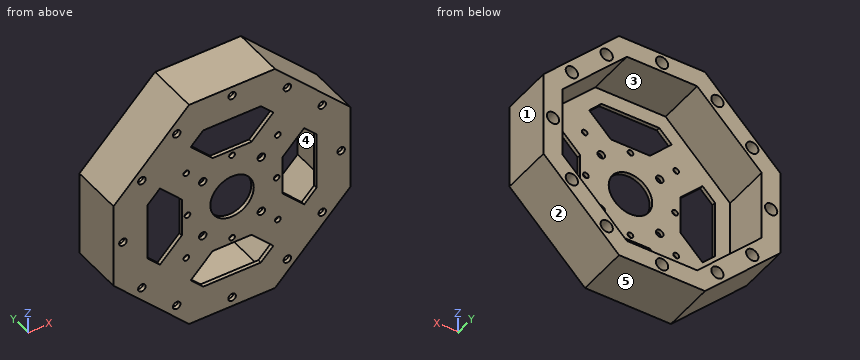
Autodesk Inventor part; units mm, degrees
ref_plane "YZ Plane" through (0, 0, 0) normal (1, 0, 0) x (0, 1, 0)
ref_plane "XZ Plane" through (0, 0, 0) normal (0, 1, 0) x (-1, 0, 0)
ref_plane "XY Plane" through (0, 0, 0) normal (0, 0, 1) x (1, 0, 0)
sketch "Sketch1" plane through (0, 0, 0) normal (0, 1, 0) x (-1, 0, 0)
  line L0 (0, 0) -> (0, 22.75)
  line L1 (40, 62.75) -> (0, 22.75)
  line L2 (40, 62.75) -> (85.5, 62.75)
  line L3 (85.5, 62.75) -> (125.5, 22.75)
  line L4 (125.5, 22.75) -> (125.5, 0)
  line L5 (0, 0) -> (0, -22.75)
  line L6 (40, -62.75) -> (0, -22.75)
  line L7 (40, -62.75) -> (85.5, -62.75)
  line L8 (85.5, -62.75) -> (125.5, -22.75)
  line L9 (125.5, -22.75) -> (125.5, 0)
  dimension "d0" = 22.75
  dimension "d3" = 45.5
  dimension "d4" = 135
extrude "Extrusion1" add sketch "Sketch1" along normal blind 2
sketch "Sketch2" plane through (0, 2, 0) normal (0, 1, 0) x (1, 0, 0)
  line L0 (-85.5, -62.75) -> (-40, -62.75)
  line L1 (-62.75, -62.75) -> (-62.75, 0)
  circle A0 centre (-62.75, 0) radius 11.5
  point P0 (0, 0)
  point P1 (-78.25, -15.5)
  point P2 (-47.25, -15.5)
  point P3 (-47.25, 15.5)
  point P4 (-78.25, 15.5)
  dimension "d7" = 23
extrude "Extrusion2" cut sketch "Sketch2" against normal blind 2
sketch "Sketch3" plane through (0, 2, 0) normal (0, 1, 0) x (1, 0, 0)
  circle A0 centre (-62.75, 0) radius 11.5
  point P0 (0, 0)
  point P1 (-78.25, -15.5)
  point P2 (-47.25, -15.5)
  point P3 (-47.25, 15.5)
  point P4 (-78.25, 15.5)
hole "Hole1" at (-78.25, 2, 15.5) at (-47.25, 2, 15.5) at (-47.25, 2, -15.5) at (-78.25, 2, -15.5) direction (0, -1, 0) diameter 4 depth 2 tip angle 118
sketch "Sketch4" plane through (0, 2, 0) normal (0, 1, 0) x (1, 0, 0)
  line L0 (-125.5, -22.75) -> (-85.5, -62.75)
  line L1 (-85.5, -62.75) -> (-125.5, -22.75)
  line L2 (-125.5, 22.75) -> (-125.5, -22.75)
  line L3 (-125.5, -22.75) -> (-125.5, 22.75)
  line L4 (-85.5, 62.75) -> (-125.5, 22.75)
  line L5 (-125.5, 22.75) -> (-85.5, 62.75)
  line L6 (-40, 62.75) -> (-85.5, 62.75)
  line L7 (-85.5, 62.75) -> (-40, 62.75)
  line L8 (0, -22.75) -> (0, 22.75)
  line L9 (-40, 62.75) -> (0, 22.75)
  line L10 (0, 22.75) -> (0, -22.75)
  line L11 (-40, -62.75) -> (0, -22.75)
  line L12 (0, -22.75) -> (-40, -62.75)
  line L13 (-85.5, -62.75) -> (-40, -62.75)
  line L14 (-40, -62.75) -> (-85.5, -62.75)
  circle A0 centre (-62.75, 0) radius 11.5
  point P0 (0, 0)
  point P1 (-62.75, -57.75)
  point P2 (-92.0542, -49.1247)
  point P3 (-110.5001, -30.6788)
  point P4 (-33.4458, -49.1247)
  point P5 (-14.9999, -30.6788)
  point P6 (-5, 0)
  point P7 (-120.5, 0)
  point P8 (-62.75, 57.75)
  point P9 (-92.0542, 49.1247)
  point P10 (-110.5001, 30.6788)
  point P11 (-33.4458, 49.1247)
  point P12 (-14.9999, 30.6788)
hole "Hole2" at (-62.75, 2, 57.75) at (-92.0542, 2, 49.1247) at (-110.5001, 2, 30.6788) at (-33.4458, 2, 49.1247) at (-14.9999, 2, 30.6788) at (-5, 2, 0) at (-120.5, 2, 0) at (-110.5001, 2, -30.6788) at (-92.0542, 2, -49.1247) at (-62.75, 2, -57.75) at (-33.4458, 2, -49.1247) at (-14.9999, 2, -30.6788) direction (0, -1, 0) diameter 4 depth 2 tip angle 118
sketch "Sketch5" plane through (0, 2, 0) normal (0, 1, 0) x (1, 0, 0)
  line L0 (-40, -62.75) -> (0, -22.75)
  line L1 (-85.5, -62.75) -> (-40, -62.75)
  line L2 (-40, -62.75) -> (-85.5, -62.75)
  line L3 (-125.5, 22.75) -> (-125.5, -22.75)
  line L4 (-85.5, -62.75) -> (-125.5, -22.75)
  line L5 (-125.5, -22.75) -> (-125.5, 22.75)
  line L6 (-85.5, 62.75) -> (-125.5, 22.75)
  line L7 (-125.5, 22.75) -> (-85.5, 62.75)
  line L8 (-40, 62.75) -> (-85.5, 62.75)
  line L9 (-85.5, 62.75) -> (-40, 62.75)
  line L10 (0, -22.75) -> (0, 22.75)
  line L11 (-40, 62.75) -> (0, 22.75)
  line L12 (0, 22.75) -> (0, -22.75)
  line L13 (0, -22.75) -> (-40, -62.75)
  line L14 (-81.3579, -52.75) -> (-44.1421, -52.75)
  line L15 (-10, -18.6079) -> (-10, 18.6079)
  line L16 (-44.1421, 52.75) -> (-81.3579, 52.75)
  line L17 (-115.5, 18.6079) -> (-115.5, -18.6079)
  line L18 (-49.1421, -18.6079) -> (-76.3579, -18.6079)
  line L19 (-81.3579, -13.6079) -> (-81.3579, 13.6079)
  line L20 (-76.3579, 18.6079) -> (-49.1421, 18.6079)
  line L21 (-44.1421, 13.6079) -> (-44.1421, -13.6079)
  line L22 (-44.1421, -13.6079) -> (-24.5711, -33.1789)
  line L23 (-49.1421, -18.6079) -> (-29.5711, -38.1789)
  line L24 (-76.3579, -18.6079) -> (-95.9289, -38.1789)
  line L25 (-81.3579, -13.6079) -> (-100.9289, -33.1789)
  line L26 (-81.3579, 13.6079) -> (-100.9289, 33.1789)
  line L27 (-76.3579, 18.6079) -> (-95.9289, 38.1789)
  line L28 (-49.1421, 18.6079) -> (-29.5711, 38.1789)
  line L29 (-44.1421, 13.6079) -> (-24.5711, 33.1789)
  line L30 (-115.5, -18.6079) -> (-100.9289, -33.1789)
  line L31 (-95.9289, -38.1789) -> (-81.3579, -52.75)
  line L32 (-44.1421, -52.75) -> (-29.5711, -38.1789)
  line L33 (-24.5711, -33.1789) -> (-10, -18.6079)
  line L34 (-10, 18.6079) -> (-24.5711, 33.1789)
  line L35 (-29.5711, 38.1789) -> (-44.1421, 52.75)
  line L36 (-91.6863, -38.1789) -> (-75.1152, -21.6079)
  line L37 (-75.1152, -21.6079) -> (-50.3848, -21.6079)
  line L38 (-50.3848, -21.6079) -> (-33.8137, -38.1789)
  line L39 (-33.8137, -38.1789) -> (-45.3848, -49.75)
  line L40 (-45.3848, -49.75) -> (-80.1152, -49.75)
  line L41 (-80.1152, -49.75) -> (-91.6863, -38.1789)
  line L42 (-81.3579, 52.75) -> (-95.9289, 38.1789)
  line L43 (-100.9289, 33.1789) -> (-115.5, 18.6079)
  line L44 (-100.9289, -28.9363) -> (-84.3579, -12.3652)
  line L45 (-84.3579, -12.3652) -> (-84.3579, 12.3652)
  line L46 (-84.3579, 12.3652) -> (-100.9289, 28.9363)
  line L47 (-100.9289, 28.9363) -> (-112.5, 17.3652)
  line L48 (-112.5, 17.3652) -> (-112.5, -17.3652)
  line L49 (-112.5, -17.3652) -> (-100.9289, -28.9363)
  line L50 (-91.6863, 38.1789) -> (-75.1152, 21.6079)
  line L51 (-75.1152, 21.6079) -> (-50.3848, 21.6079)
  line L52 (-50.3848, 21.6079) -> (-33.8137, 38.1789)
  line L53 (-33.8137, 38.1789) -> (-45.3848, 49.75)
  line L54 (-45.3848, 49.75) -> (-80.1152, 49.75)
  line L55 (-80.1152, 49.75) -> (-91.6863, 38.1789)
  line L56 (-41.1421, -12.3652) -> (-41.1421, 12.3652)
  line L57 (-41.1421, 12.3652) -> (-24.5711, 28.9363)
  line L58 (-24.5711, 28.9363) -> (-13, 17.3652)
  line L59 (-13, 17.3652) -> (-13, -17.3652)
  line L60 (-13, -17.3652) -> (-24.5711, -28.9363)
  line L61 (-24.5711, -28.9363) -> (-41.1421, -12.3652)
  line L62 (-73.0442, -26.6079) -> (-84.6152, -38.1789)
  line L63 (-84.6152, -38.1789) -> (-78.0442, -44.75)
  line L64 (-78.0442, -44.75) -> (-47.4558, -44.75)
  line L65 (-47.4558, -44.75) -> (-40.8848, -38.1789)
  line L66 (-40.8848, -38.1789) -> (-52.4558, -26.6079)
  line L67 (-52.4558, -26.6079) -> (-73.0442, -26.6079)
  line L68 (-100.9289, -21.8652) -> (-89.3579, -10.2942)
  line L69 (-89.3579, -10.2942) -> (-89.3579, 10.2942)
  line L70 (-89.3579, 10.2942) -> (-100.9289, 21.8652)
  line L71 (-100.9289, 21.8652) -> (-107.5, 15.2942)
  line L72 (-107.5, 15.2942) -> (-107.5, -15.2942)
  line L73 (-107.5, -15.2942) -> (-100.9289, -21.8652)
  line L74 (-73.0442, 26.6079) -> (-84.6152, 38.1789)
  line L75 (-84.6152, 38.1789) -> (-78.0442, 44.75)
  line L76 (-78.0442, 44.75) -> (-47.4558, 44.75)
  line L77 (-47.4558, 44.75) -> (-40.8848, 38.1789)
  line L78 (-40.8848, 38.1789) -> (-52.4558, 26.6079)
  line L79 (-52.4558, 26.6079) -> (-73.0442, 26.6079)
  line L80 (-36.1421, 10.2942) -> (-36.1421, -10.2942)
  line L81 (-36.1421, -10.2942) -> (-24.5711, -21.8652)
  line L82 (-24.5711, -21.8652) -> (-18, -15.2942)
  line L83 (-18, -15.2942) -> (-18, 15.2942)
  line L84 (-18, 15.2942) -> (-24.5711, 21.8652)
  line L85 (-24.5711, 21.8652) -> (-36.1421, 10.2942)
  point P0 (0, 0)
  dimension "d39" = 3
  dimension "d40" = 3
  dimension "d41" = 3
  dimension "d42" = 3
  dimension "d59" = 7.0711
  dimension "d60" = 7.0711
  dimension "d61" = 5
  dimension "d62" = 5
  dimension "d63" = 5
  dimension "d64" = 5
extrude "Extrusion3" cut sketch "Sketch5" against normal blind 2 contours L67 L66 L65 L64 L63 L62 | L73 L72 L71 L70 L69 L68 | L74 L75 L76 L77 L78 L79 | L85 L84 L83 L82 L81 L80
sketch "Sketch6" plane through (0, 2, 0) normal (0, 1, 0) x (1, 0, 0)
  line L0 (-85.5, -62.75) -> (-40, -62.75)
  line L1 (-125.5, -22.75) -> (-85.5, -62.75)
  line L2 (-40, -62.75) -> (-85.5, -62.75)
  line L3 (-85.5, -62.75) -> (-125.5, -22.75)
  line L4 (-85.5, 62.75) -> (-125.5, 22.75)
  line L5 (-125.5, -22.75) -> (-125.5, 22.75)
  line L6 (-125.5, 22.75) -> (-85.5, 62.75)
  line L7 (-40, 62.75) -> (-85.5, 62.75)
  line L8 (-85.5, 62.75) -> (-40, 62.75)
  line L9 (0, -22.75) -> (0, 22.75)
  line L10 (-40, 62.75) -> (0, 22.75)
  line L11 (0, 22.75) -> (0, -22.75)
  line L12 (-40, -62.75) -> (0, -22.75)
  line L13 (0, -22.75) -> (-40, -62.75)
  line L14 (-115.5, 18.6079) -> (-115.5, -18.6079)
  line L15 (-115.5, -18.6079) -> (-81.3579, -52.75)
  line L16 (-81.3579, -52.75) -> (-44.1421, -52.75)
  line L17 (-44.1421, -52.75) -> (-10, -18.6079)
  line L18 (-10, -18.6079) -> (-10, 18.6079)
  line L19 (-10, 18.6079) -> (-44.1421, 52.75)
  line L20 (-44.1421, 52.75) -> (-81.3579, 52.75)
  line L21 (-81.3579, 52.75) -> (-115.5, 18.6079)
  circle A0 centre (-62.75, -57.75) radius 2
  circle A1 centre (-62.75, -57.75) radius 3.25
  circle A2 centre (-92.0542, -49.1247) radius 2
  circle A3 centre (-92.0542, -49.1247) radius 3.25
  circle A4 centre (-110.5001, -30.6788) radius 2
  circle A5 centre (-110.5001, -30.6788) radius 3.25
  circle A6 centre (-120.5, 0) radius 2
  circle A7 centre (-120.5, 0) radius 3.25
  circle A8 centre (-110.5001, 30.6788) radius 2
  circle A9 centre (-110.5001, 30.6788) radius 3.25
  circle A10 centre (-92.0542, 49.1247) radius 2
  circle A11 centre (-92.0542, 49.1247) radius 3.25
  circle A12 centre (-62.75, 57.75) radius 2
  circle A13 centre (-62.75, 57.75) radius 3.25
  circle A14 centre (-33.4458, 49.1247) radius 2
  circle A15 centre (-33.4458, 49.1247) radius 3.25
  circle A16 centre (-14.9999, 30.6788) radius 2
  circle A17 centre (-14.9999, 30.6788) radius 3.25
  circle A18 centre (-5, 0) radius 2
  circle A19 centre (-5, 0) radius 3.25
  circle A20 centre (-14.9999, -30.6788) radius 2
  circle A21 centre (-14.9999, -30.6788) radius 3.25
  circle A22 centre (-33.4458, -49.1247) radius 2
  circle A23 centre (-33.4458, -49.1247) radius 3.25
  point P0 (0, 0)
  dimension "d45" = 10
  dimension "d46" = 6.5
  dimension "d47" = 6.5
  dimension "d48" = 6.5
  dimension "d49" = 6.5
extrude "Extrusion4" add sketch "Sketch6" along normal blind 25.4 contours L1 L5 L4 L7 L10 L9 L12 L0
sketch "Sketch8" plane through (0, 0, 0) normal (0, -1, 0) x (1, 0, 0)
  line L0 (-52.4558, 26.6079) -> (-73.0442, 26.6079)
  circle A0 centre (-62.75, 0) radius 11.5
  circle A1 centre (-62.75, 0) radius 11.5
  line L1 (-73.0442, 26.6079) -> (-84.6152, 38.1789)
  line L2 (-100.9289, 21.8652) -> (-89.3579, 10.2942)
  line L3 (-36.1421, -10.2942) -> (-36.1421, 10.2942)
  line L4 (-73.0442, -26.6079) -> (-52.4558, -26.6079)
  line L5 (-89.3579, 10.2942) -> (-89.3579, -10.2942)
  point P0 (0, 0)
  point P1 (-39.1421, 0)
  point P2 (-62.75, -23.6079)
  point P3 (-86.3579, 0)
  point P4 (-62.75, 23.6079)
  point P5 (-86.9865, 24.2366)
  point P6 (-38.5134, 24.2365)
  point P7 (-38.5135, -24.2366)
  point P8 (-86.9866, -24.2365)
  dimension "d82" = 3
  dimension "d83" = 3
  dimension "d84" = 3
  dimension "d85" = 3
hole "Hole4" at (-39.1421, 0, 0) at (-62.75, 0, -23.6079) at (-86.3579, 0, 0) at (-62.75, 0, 23.6079) at (-86.9865, 0, 24.2366) at (-38.5134, 0, 24.2365) at (-38.5135, 0, -24.2366) at (-86.9866, 0, -24.2365) direction (0, 1, 0) diameter 3 depth 2 tip angle 118
properties part number "Base_Lid"
Build history of the part. All positions in model axes, mm. Face numbers are marked on the shaded views. A direction names the side the tool comes from. Give positions to 0.01 mm unless a question says otherwise; leave off trailing zeros. Loops run counter-clockwise (first coordinate to the right, second up) from the corner with the lowest first, then second, coordinate; pieces in that order, holes last. Notation, with made-up numbers: (17.5, 66) - (58.5, 66) arc R8 cw to (58.5, 76) - close; hole circle Ø8 at (61, -32.75). An arc over 180 degrees is marked (long way). Write item = value, one per line. Start each with the question number.
1) Band-saw the part on C-C on y = 14.5. Count the separate pieces of the cut face and the enclosed holes in it, plus the area to 3 significant figures.
2) Tool access for the marked faces 4 and 5: list every direction of +Z, -Z, +X, -X, +Y, -Y with a clear straight run to the whole face (end or side of a thin tool).
3) Drop flat-ended pins along their axis: pin 1 Ø6 at (x, z) = (-51.5, 10) entering from -Y; pin 2 Ø2 at (x, z) = (-33.5, -48.5) entering from +Y; pin 3 Ø8 at (x, z) = (-28.5, -16.5) entering from +Y; pin 4 Ø1 at (y, z) = (22, -50) entering from -X. Give the stop position or say it passes through.
4) Probe probe 1 along X at (y, z) = (25.75, -17); probe 2 along Z at (x, y) = (-45, 3.5); probe 3 along Z at (x, y) = (-12, 2.75). List the from-to ranges inside material, lowest first. Write a range as from..to.
5) Pull direction Z, two halves, no side cores. Call the marked faces 1, 2 and 3: +Z half, -Z half, draft (parallel to the pull), parting line (faces both ways), or undercut.
6) Band-saw the part on A-A on x = -120.5. Give the cut face in (y, z).
7) Band-saw the part on B-B on z = 57.75. Give the cut face in (x, y).
Final values:
q1.separate_pieces = 1
q1.enclosed_holes = 13
q1.area = 3,350 mm²
q2.face_4 = +Y
q2.face_5 = -Z, +X, -X, +Y, -Y
q3.pin_1 = 0
q3.pin_2 = through
q3.pin_3 = 2
q3.pin_4 = -98.75
q4.probe_1 = -125.5..-115.5, -10..0
q4.probe_2 = -62.75..-52.75, 52.75..62.75
q4.probe_3 = -34.75..-31.93, -29.43..-20.61, 20.61..29.43, 31.93..34.75
q5.face_1 = draft
q5.face_2 = -Z half
q5.face_3 = undercut
q6.outline = (0, -27.75) - (27.4, -27.75) - (27.4, -3.25) - (2, -3.25) - (2, -2) - (0, -2) - close; (0, 2) - (2, 2) - (2, 3.25) - (27.4, 3.25) - (27.4, 27.75) - (0, 27.75) - close
q7.outline = (-90.5, 0) - (-64.75, 0) - (-64.75, 2) - (-66, 2) - (-66, 27.4) - (-90.5, 27.4) - close; (-60.75, 0) - (-35, 0) - (-35, 27.4) - (-59.5, 27.4) - (-59.5, 2) - (-60.75, 2) - close
